Drawing for the job (mm, zero at the part's lowest x, y, z). A direction names the side the tool comes from. Round coordinates to 2 decimals unless told otherwise and drop trailing zeros. Loops run counter-clockwise (first coordinate to the right, second up) from the corner with the lowest first, then second, coordinate; pieces in that order, holes last. Notation, with made-up numbers: M 31,25.5 L 72,25.5 A29 ccw 72,47.5 Z; hole C -36.75,13 d9. An arc over 180 degrees is marked long. Answer in a Markdown table with one row per item.
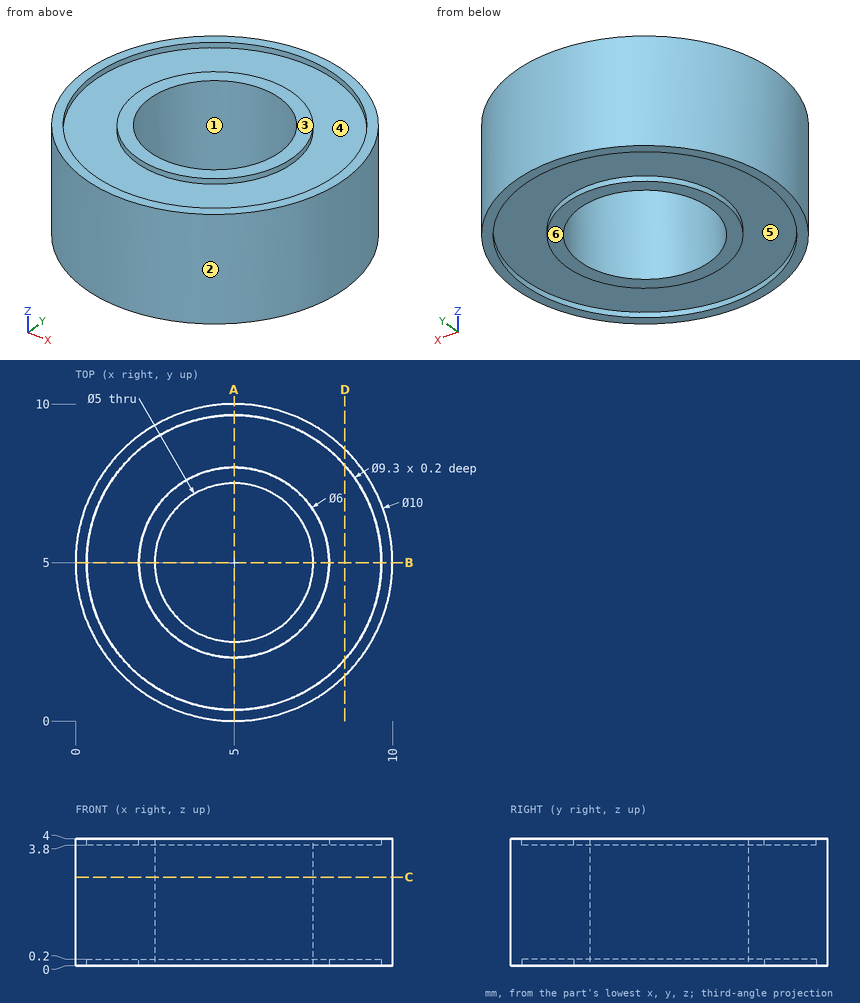
1. Tool access for the marked faces 4, 5 and 6: list every direction of +Z, -Z, +X, -X, +Y, -Y with a clear straight run to the whole face (end or side of a thin tool).
Verdict:
| item | result |
|---|---|
| face 4 | +Z |
| face 5 | -Z |
| face 6 | -Z, +X, -X, +Y, -Y |
2. Saw through at D-D (x = 8.5). Write the cut outline in (y, z), and give its area (3 significant figures).
Verdict:
| item | result |
|---|---|
| outline | M 1.43,0 L 1.94,0 L 1.94,0.2 L 8.06,0.2 L 8.06,0 L 8.57,0 L 8.57,4 L 8.06,4 L 8.06,3.8 L 1.94,3.8 L 1.94,4 L 1.43,4 Z |
| area | 26.1 mm² |
3. Wall check: probe 1 along Y at (x, z) = (5, 3.9); probe 2 along Z at (x, y) = (5.25, 8.5); probe 3 along Y at (x, z) = (5, 2). Give the ranges that are in metal, low to high.
Verdict:
| item | result |
|---|---|
| probe 1 | y = 0 to 0.35, 2 to 2.5, 7.5 to 8, 9.65 to 10 |
| probe 2 | z = 0.2 to 3.8 |
| probe 3 | y = 0 to 2.5, 7.5 to 10 |
4. Saw through at C-C (z = 2.8). Write the cut outline in (x, y), and give its area (3 significant figures).
Verdict:
| item | result |
|---|---|
| outline | C 5,5 d10; hole C 5,5 d5 |
| area | 58.9 mm² |
5. Mould opens along Y. For the marked faces 1, 2 and 3 say: +Y half, -Y half, draft (parallel to the pull), parting line (faces both ways), or undercut.
Verdict:
| item | result |
|---|---|
| face 1 | undercut |
| face 2 | parting line |
| face 3 | draft |
6. Pin check, flat tips, straight feed: pin 1 (1 mm diameter, centred on x = 7.5, z = 1.5, fed in from +Y); pin 2 (1.5 mm diameter, centred on y = 7.5, z = 3.5, fed in from -X). Stop position of each tip, or through.
Verdict:
| item | result |
|---|---|
| pin 1 | stops at y = 9.58 |
| pin 2 | stops at x = 0.32 |
7. Saw through at A-A (x = 5). Write the cut outline in (y, z), and give its area (3 significant figures).
Verdict:
| item | result |
|---|---|
| outline | M 0,0 L 0.35,0 L 0.35,0.2 L 2,0.2 L 2,0 L 2.5,0 L 2.5,4 L 2,4 L 2,3.8 L 0.35,3.8 L 0.35,4 L 0,4 Z; M 7.5,0 L 8,0 L 8,0.2 L 9.65,0.2 L 9.65,0 L 10,0 L 10,4 L 9.65,4 L 9.65,3.8 L 8,3.8 L 8,4 L 7.5,4 Z |
| area | 18.7 mm² |
